Verification items for the finished model (mm, model axes). Face numbers are marked on the shaded views. Give positions to 0.01 mm unless a question says otherwise; leave off trailing zeros. Loops run counter-clockwise (first coordinate to the right, second up) from the corner with the lowest first, then second, coordinate; pieces in that order, holes last. Notation, with made-up numbers: (-26, -35) - (17, -35) arc R32 cw to (17, 2) - close; hole circle Ø3 at (14, 60.5). An arc over 180 degrees is marked (long way). Answer in a Markdown table with one row per item.
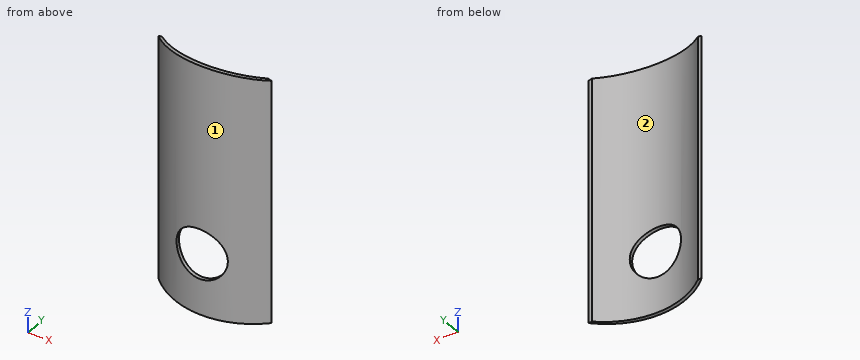
```python
from build123d import *

# Parameters (mm, degrees)
BOSS_EXTRUDE1_DEPTH = 8
FILLET1_R           = 0.5
SKETCH2_R           = 3.5
CUT_EXTRUDE1_DEPTH  = 22.5
SKETCH5_OUTSIDE_W   = 25.862
SKETCH5_OUTSIDE_H   = 17.862
CUT_EXTRUDE2_DEPTH  = 39.5
SKETCH6_OUTSIDE_W   = 25.128
SKETCH6_OUTSIDE_H   = 12.878
CUT_EXTRUDE3_DEPTH  = 39.5


with BuildPart() as part:
    # Sketch1 → Boss-Extrude1 (new body)
    with BuildSketch(Plane(origin=(0, 0, 0), x_dir=(1, 0, 0), z_dir=(0, 1, 0))):
        with BuildLine():
            Line((8, -16.5), (8, 17.5))
            Line((8, 17.5), (-8, 17.5))
            Line((-8, 17.5), (-8, -16.5))
            ThreePointArc((-8, -16.5), (0, -17.5), (8, -16.5))
        make_face()
    extrude(amount=BOSS_EXTRUDE1_DEPTH)

    # Fillet1
    fillet1_edges = [part.edges().sort_by_distance(p)[0] for p in [
        (-8, 4, -17.5),
        (8, 4, -17.5),
        (8, 4, 16.5),
        (-8, 4, 16.5),
    ]]
    fillet(fillet1_edges, radius=FILLET1_R)

    # Sketch2 → Cut-Extrude1 (cut)
    with BuildSketch(Plane(origin=(0, 8, 0), x_dir=(1, 0, 0), z_dir=(0, 1, 0))):
        with Locations(Location((0, 9, 0), (0, 0, 270))):
            Circle(SKETCH2_R)
    extrude(amount=-CUT_EXTRUDE1_DEPTH, mode=Mode.SUBTRACT)

    # Sketch5 outside → Cut-Extrude2 (cut, symmetric)
    with BuildSketch(Plane(origin=(0, 0, -17.5), x_dir=(-1, 0, 0), z_dir=(0, 0, -1))):
        with Locations((0, 4)):
            Rectangle(SKETCH5_OUTSIDE_W, SKETCH5_OUTSIDE_H)
        with BuildLine():
            Line((0, 8), (-7.725, 8))
            ThreePointArc((-7.725, 8), (0, 4.8), (7.725, 8))
            Line((7.725, 8), (0, 8))
        make_face(mode=Mode.SUBTRACT)
    extrude(amount=CUT_EXTRUDE2_DEPTH, both=True, mode=Mode.SUBTRACT)

    # Sketch6 outside → Cut-Extrude3 (cut, symmetric)
    with BuildSketch(Plane(origin=(0, 0, -17.5), x_dir=(-1, 0, 0), z_dir=(0, 0, -1))):
        with Locations((0, 6.4)):
            Rectangle(SKETCH6_OUTSIDE_W, SKETCH6_OUTSIDE_H)
        with BuildLine():
            Line((-7.725, 8), (-7.225, 8))
            ThreePointArc((-7.225, 8), (0, 5.320884761), (7.225, 8))
            Line((7.225, 8), (7.725, 8))
            ThreePointArc((7.725, 8), (0, 4.820884761), (-7.725, 8))
        make_face(mode=Mode.SUBTRACT)
    extrude(amount=CUT_EXTRUDE3_DEPTH, both=True, mode=Mode.SUBTRACT)


solid = part.part
```
Q1. Sectioned sample at C-C (z = 6). Record the cut outline in (x, y) (3 decimals), and give its area (3 significant figures).
Completed:
| item | result |
|---|---|
| outline | (-7.725, 8) arc R10.975 ccw to (7.725, 8) - (7.225, 8) arc R11.082 cw to (-7.225, 8) - close |
| area | 7.32 mm^2 |
Q2. Sectioned sample at B-B (y = 7.2). Record the cut outline in (x, z), and give its area (3 significant figures).
Completed:
| item | result |
|---|---|
| outline | (-6.82, -17.5) - (-6.17, -17.5) - (-6.17, 16.91) arc R32.5 ccw to (-6.82, 16.78) - close; (6.17, -17.5) - (6.82, -17.5) - (6.82, 16.78) arc R32.5 ccw to (6.17, 16.91) - close |
| area | 44.6 mm^2 |
Q3. Go/stop test with flat-tipped pins: P1, Ø1, axis at y = 5.5, z = -9.5, coming from the -X side; P2, Ø3, axis at x = 3.5, z = 10.5, coming from the +Y side. Record where each tip stops, or that it passes through.
Completed:
| item | result |
|---|---|
| P1 | x = -4.95 |
| P2 | y = 6.51 |
Q4. Sectioned sample at D-D (x = 5.75). Record the cut outline in (y, z).
Completed:
| item | result |
|---|---|
| outline | (6.45, -17.5) - (6.93, -17.5) - (6.93, 16.99) - (6.45, 16.99) - close |
Q5. Sectioned sample at A-A (x = 0). Record the cut outline in (y, z), and give its area (3 significant figures).
Completed:
| item | result |
|---|---|
| outline | (4.82, -17.5) - (5.32, -17.5) - (5.32, -12.5) - (4.82, -12.5) - close; (4.82, -5.5) - (5.32, -5.5) - (5.32, 17.5) - (4.82, 17.5) - close |
| area | 14.0 mm^2 |
Q6. Draft check along X on the marked faces 1 and 2. Enter one of: +X half, -X half, draft (parallel to the pull), parting line (faces both ways), or undercut.
Completed:
| item | result |
|---|---|
| face 1 | parting line |
| face 2 | undercut |
Q7. Thickness scan on line 1 (Z direction, x = 0, y = 5.25); line 2 (X direction, y = 7.25, z = -12); line 3 (Z direction, x = -2, y = 5.2). Record the ranges inside material, lowest first.
Completed:
| item | result |
|---|---|
| line 1 | -17.5 to -12.5, -5.5 to 17.5 |
| line 2 | -6.89 to -6.25, 6.25 to 6.89 |
| line 3 | -17.5 to -11.87, -6.13 to 17.44 |
